Check sheet for the modelled part. Datum: model origin and axes. Units: mm. Face numbers are marked on the shaded views. A direction names the side the tool comes from. Give positions to 0.01 mm unless a question says otherwise; leave off trailing zeros. Loops run counter-clockwise (first coordinate to the right, second up) from the corner with the lowest first, then second, coordinate; pieces in that order, holes last.
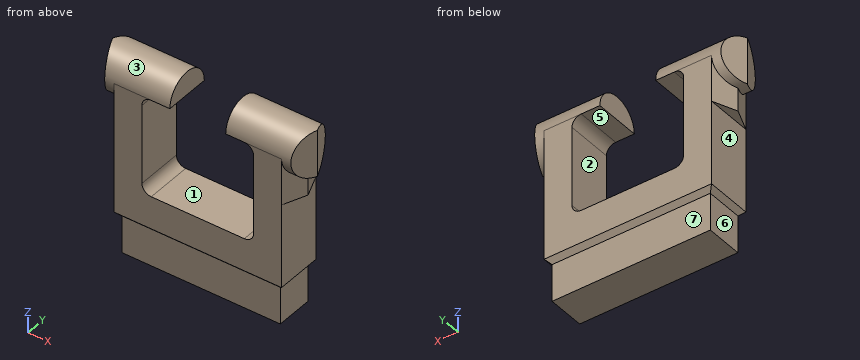
```python
from build123d import *

# Parameters (mm, degrees)
F2_DEPTH    = 2.5
F3_DEPTH    = 10
F4_DEPTH    = 3
F5_DEPTH    = 6
F6_T1_DEPTH = 5
F8_DEPTH    = 14
F9_DEPTH    = 9
F10_DEPTH   = 1
F11_DEPTH   = 16.5
F12_FACE_W  = 18
F12_FACE_H  = 5
F13_DEPTH   = 0.5
F13_TAPER   = 45
F14_DEPTH   = 4


# Not quite as in the source:
# - a fillet or chamfer that OpenCascade refuses, or shapes differently, is made with other operations: its cross-section is extruded or revolved along the edge and cut away or added


with BuildPart() as f2:
    # F0 (on Front) → F2 (new body, symmetric)
    with BuildSketch(Plane.XZ):
        Polygon((0, 3.5), (0, 0), (9, 0), (9, 14), (6, 14), (6, 3.5), align=None)
    extrude(amount=F2_DEPTH, both=True)

    # F1 (on Right) → F3 (join)
    with BuildSketch(Plane.YZ):
        with BuildLine():
            Line((-2.5, 14), (2.5, 14))
            ThreePointArc((2.5, 14), (0, 16.5), (-2.5, 14))
        make_face()
        with BuildLine():
            ThreePointArc((-2.5, 14), (0, 11.5), (2.5, 14))
            Line((2.5, 14), (-2.5, 14))
        make_face()
    extrude(amount=F3_DEPTH)

    # F1 (on Right) → F4 (cut)
    with BuildSketch(Plane.YZ):
        with BuildLine():
            Line((-2.5, 14), (2.5, 14))
            ThreePointArc((2.5, 14), (0, 16.5), (-2.5, 14))
        make_face()
        with BuildLine():
            ThreePointArc((-2.5, 14), (0, 11.5), (2.5, 14))
            Line((2.5, 14), (-2.5, 14))
        make_face()
    extrude(amount=F4_DEPTH, mode=Mode.SUBTRACT)

    # F1 (on Right) → F5 (cut)
    with BuildSketch(Plane.YZ):
        with BuildLine():
            ThreePointArc((-2.5, 14), (0, 11.5), (2.5, 14))
            Line((2.5, 14), (-2.5, 14))
        make_face()
    extrude(amount=F5_DEPTH, mode=Mode.SUBTRACT)

    # F6: fillet of radius 1 on 2 edges, made by hand

    # F6_s2 → F6_t1 (join)
    with BuildSketch(Plane.XZ.offset(-2.5)):
        with BuildLine():
            ThreePointArc((6, 13), (5.7071067812, 13.7071067812), (5, 14))
            Line((5, 14), (6, 14))
            Line((6, 14), (6, 13))
        make_face()
        with BuildLine():
            ThreePointArc((5, 3.5), (5.7071067812, 3.7928932188), (6, 4.5))
            Line((6, 4.5), (6, 3.5))
            Line((6, 3.5), (5, 3.5))
        make_face()
    extrude(amount=F6_T1_DEPTH)

    # F7 (on Top) → F8 (join)
    with BuildSketch(Plane.XY):
        Polygon((9, 2.5), (9, -2.5), (10, 0), align=None)
    extrude(amount=F8_DEPTH)

    # F7 (on Top) → F9 (cut)
    with BuildSketch(Plane.XY):
        Polygon((9, 2.5), (9, -2.5), (10, 0), align=None)
    extrude(amount=F9_DEPTH, mode=Mode.SUBTRACT)

    # F10 (add): a face of the model
    f10_faces = [f2.faces().sort_by_distance(p)[0] for p in [
        (10, -1.717766953, 12.282233047),
    ]]
    extrude(f10_faces, amount=F10_DEPTH)

    # F7 (on Top) → F11 (cut)
    with BuildSketch(Plane.XY):
        Polygon((11, 0), (10, -2.5), (11.5, -2.5), (11.5, 2.5), (10, 2.5), align=None)
    extrude(amount=F11_DEPTH, mode=Mode.SUBTRACT)

    # F12: F2 across face


with BuildPart() as f2_1:
    add(f2.part)
    add(f2.part.mirror(Plane(origin=(0, 0, 1.75), x_dir=(0, -1, 0), z_dir=(-1, 0, 0))))

    # F12_face (on face) → F13 (join)
    with BuildSketch(Plane(origin=(0, 0, 0), x_dir=(1, 0, 0), z_dir=(0, 0, -1))):
        Rectangle(F12_FACE_W, F12_FACE_H)
    extrude(amount=F13_DEPTH, taper=F13_TAPER)

    # F14 (add): a face of the model
    f14_faces = [f2_1.faces().sort_by_distance(p)[0] for p in [
        (0, 0, -0.5),
    ]]
    extrude(f14_faces, amount=F14_DEPTH)


solid = f2_1.part
```
(1) Section check C-C on z = 0.75. Record the boundary of the cut face in (x, y), plus the area to 3 significant figures.
(2) Material ranges on line 1 (X direction, y = -0.4, z = 6); line 2 (X direction, y = 0.1, z = 11); line 3 (Z direction, x = 2.5, y = 1.7), recorded low to high.
(3) Section check D-D on z = -2.25. Record the boundary of the cut face in (x, y).
(4) Section check A-A on z = 6.5. Record the boundary of the cut face in (x, y), plus the area to 3 significant figures.
(5) Access from +Z, -Z, +X, -X, +Y, -Y to the whole of each face (thin tool, end or side, straight path). Record for the marked faces 5, 6 and 7.
(6) Release check for a two-part mould opening along Z. For the marked faces 1, 2, 3 and 4 record: pulls with the +Z half, pulls with the -Z half, needs draft (parallel to the pull), parting line crosses it, or undercut.
(7) Section check B-B on z = 10.25. Record the boundary of the cut face in (x, y), plus the area to 3 significant figures.
(8) Gauge pin test, flat ends, axial feed: pin 1 Ø1.2 at (y, z) = (-1, -2.5) entering from -X; pin 2 Ø2.5 at (y, z) = (-0.5, 3) entering from -X; pin 3 Ø2 at (x, z) = (-3.5, -2) entering from +Y. Record the tip position at first contact, or that the pin passes through.
Computed values:
1. outline: (-9, -2.5) - (9, -2.5) - (9, 2.5) - (-9, 2.5) - close
1. area: 90.0 mm2
2. line 1: x = -9 to -6, 6 to 9
2. line 2: x = -9.96 to -6, 6 to 9.96
2. line 3: z = -4.5 to 3.5
3. outline: (-8.5, -2) - (8.5, -2) - (8.5, 2) - (-8.5, 2) - close
4. outline: (-9, -2.5) - (-6, -2.5) - (-6, 2.5) - (-9, 2.5) - close; (6, -2.5) - (9, -2.5) - (9, 2.5) - (6, 2.5) - close
4. area: 30.0 mm2
5. face 5: +Y, -Y
5. face 6: -Z, -X, +Y, -Y
5. face 7: -Z, +X, -X, +Y
6. face 1: undercut
6. face 2: undercut
6. face 3: parting line crosses it
6. face 4: needs draft
7. outline: (-10, 0) - (-9, -2.5) - (-6, -2.5) - (-6, 2.5) - (-9, 2.5) - close; (6, -2.5) - (9, -2.5) - (10, 0) - (9, 2.5) - (6, 2.5) - close
7. area: 35.0 mm2
8. pin 1: stops at x = -8.5
8. pin 2: stops at x = -9
8. pin 3: stops at y = 2
